Autodesk Inventor part; units mm, degrees
ref_plane "YZ Plane" through (0, 0, 0) normal (1, 0, 0) x (0, 1, 0)
ref_plane "XZ Plane" through (0, 0, 0) normal (0, 1, 0) x (-1, 0, 0)
ref_plane "XY Plane" through (0, 0, 0) normal (0, 0, 1) x (1, 0, 0)
sketch "Sketch2" plane through (0, 0, 0) normal (0, 1, 0) x (-1, 0, 0)
  line L0 (-20, 20) -> (20, 20)
  line L1 (20, 20) -> (20, -20)
  line L2 (20, -20) -> (-20, -20)
  line L3 (-20, -20) -> (-20, 20)
  circle A0 centre (10, 10) radius 7
  circle A1 centre (10, -10) radius 7
  circle A2 centre (-10, -10) radius 7
  circle A3 centre (-10, 10) radius 7
  point P0 (0, 0)
extrude "Extrusion1" add sketch "Sketch2" along normal blind 5 and the other way blind 10
extrude "Extrusion2" add sketch "Sketch2" along normal blind 10 and the other way blind 5 contours A0 | A1 | A2 | A3
fillet "Fillet1" radius 0.5 4 edges at (-3, 10, 10) (-3, 10, -10) (17, 10, -10) (17, 10, 10)
properties part number "Tercer examen. Cubo LEGO. Villegas"
Work out the finished part from the listing and answer in its coordinate system (mm). A direction names the side the tool comes from. Give positions to 0.01 mm unless a question says otherwise; leave off trailing zeros. Order: outer loops, then holes, each group sorted by start corner. A loop starts at its lowest first (then second) coordinate and runs counter-clockwise, first axis right, second up. Notation, with made-up numbers: (74, 49) -> (101, 49) arc R16 cw to (101, 54) -> close; hole circle Ø1 at (-11, -39). An arc over 180 degrees is marked (long way). Answer as a JSON object with one key per item and string values. Group by question number.
1. Section C-C on z = -10 is taken. Determine the outline of the cut face in (x, y), plus the area to 3 significant figures.
2. Consider line 1 along Z through (x, y) = (10, -8.2); line 2 along X through (y, z) = (-6.5, 12.5); line 3 along Y through (x, z) = (-4.5, 2.5). Determine where each line is inside the solid, lowest interval first. Write a range as [from, to].
3. Section B-B on x = -10 is taken. Determine the outline of the cut face in (y, z), plus the area to 3 significant figures.
4. Flat-ended cylindrical pins translate along their axes: pin 1 Ø7 at (x, z) = (-8, -9.5) entering from -Y; pin 2 Ø3 at (x, z) = (2, 14) entering from +Y. Find the tip coordinate at first contact, or state that the pin passes through.
5. The mould has two halves that part along X. Classify faces 1 (the cylindrical face through (-16.466, -7.535, -7.319)), 2 (the flat face through (0, -10, 0)), 3 (the flat face through (20, -3, 0)): released by +X, released by -X, zero draft, split by the parting line, or undercut.
6. Section A-A on y = 8.75 is taken. Determine the outline of the cut face in (x, z).
7. Section D-D on z = 1.5 is taken. Determine the outline of the cut face in (x, y), plus the area to 3 significant figures.
8. A tool of negligible diameter and unlimited length cuts with its end or side. For faces 4 (the flat face through (10, 10, 10)), 5 (the cylindrical face through (3.534, -7.535, 12.681)), 6 (the cylindrical face through (6.77, 7.22, -3.79)), from which of +Z, -Z, +X, -X, +Y, -Y can it reach the whole face along a straight path? Write none if from no direction.
Result sheet:
{
 "1": {"outline": "(-20, -10) -> (-17, -10) -> (-17, -5) -> (-3, -5) -> (-3, -10) -> (3, -10) -> (3, -5) -> (17, -5) -> (17, -10) -> (20, -10) -> (20, 5) -> (17, 5) -> (17, 9.5) arc R0.5 ccw to (16.5, 10) -> (3.5, 10) arc R0.5 ccw to (3, 9.5) -> (3, 5) -> (-3, 5) -> (-3, 9.5) arc R0.5 ccw to (-3.5, 10) -> (-16.5, 10) arc R0.5 ccw to (-17, 9.5) -> (-17, 5) -> (-20, 5) -> close", "area": "600 mm^2"},
 "2": {"line 1": "z = [-20, -17], [-3, 3], [17, 20]", "line 2": "x = [-20, -16.54], [-3.46, 3.46], [16.54, 20]", "line 3": "y = [-10, 5]"},
 "3": {"outline": "(-10, -20) -> (5, -20) -> (5, -17) -> (9.5, -17) arc R0.5 ccw to (10, -16.5) -> (10, -3.5) arc R0.5 ccw to (9.5, -3) -> (5, -3) -> (5, 3) -> (9.5, 3) arc R0.5 ccw to (10, 3.5) -> (10, 16.5) arc R0.5 ccw to (9.5, 17) -> (5, 17) -> (5, 20) -> (-10, 20) -> (-10, 17) -> (-5, 17) -> (-5, 3) -> (-10, 3) -> (-10, -3) -> (-5, -3) -> (-5, -17) -> (-10, -17) -> close", "area": "600 mm^2"},
 "4": {"pin 1": "stops at y = -5", "pin 2": "stops at y = 5"},
 "5": {"face 1": "undercut", "face 2": "zero draft", "face 3": "released by +X"},
 "6": {"outline": "circle Ø14 at (-10, -10); circle Ø14 at (-10, 10); circle Ø14 at (10, -10); circle Ø14 at (10, 10)"},
 "7": {"outline": "(-20, -10) -> (20, -10) -> (20, 5) -> (-20, 5) -> close", "area": "600 mm^2"},
 "8": {"face 4": "+Z, -Z, +X, -X, +Y", "face 5": "-Y", "face 6": "+Y"}
}
